Source: CAD feature listing. Evaluate the final solid. Frame: model axes, mm. Face numbers are marked on the shaded views. A direction names the side the tool comes from. Give positions to 0.01 mm unless a question says otherwise; leave off trailing zeros. Write each loop counter-clockwise with the first axis right and the second up, starting at its lowest first coordinate (ties: lowest second). Pieces come first, ordered by that corner, then holes. Notation, with made-up numbers: (43.5, 17.25) -> (69.5, 17.25) arc R24 ccw to (69.5, 48.25) -> close; hole circle Ø2 at (-28, 47.25). An arc over 180 degrees is marked (long way). Write item = value, one per line.
Autodesk Inventor part; units mm, degrees
ref_plane "YZ Plane" through (0, 0, 0) normal (1, 0, 0) x (0, 1, 0)
ref_plane "XZ Plane" through (0, 0, 0) normal (0, 1, 0) x (-1, 0, 0)
ref_plane "XY Plane" through (0, 0, 0) normal (0, 0, 1) x (1, 0, 0)
sketch "Sketch1" plane through (0, 0, 0) normal (0, 0, 1) x (1, 0, 0)
  circle A0 centre (0, 0) radius 1.7526
  dimension "d0" = 3.5052
extrude "Extrusion1" add sketch "Sketch1" along normal blind 31.75
sketch "Sketch2" plane through (0, 0, 0) normal (0, 0, -1) x (-1, 0, 0)
  circle A0 centre (0, 0) radius 1.7526 construction
  circle A1 centre (0, 0) radius 2.8702
  dimension "d3" = 5.7404
extrude "Extrusion2" add sketch "Sketch2" along normal blind 3.5052
sketch "Sketch3" plane through (0, 0, -3.5052) normal (0, 0, -1) x (-1, 0, 0)
  circle A0 centre (0, 0) radius 2.8702
  line L0 (0, 1.604) -> (1.3891, 0.802)
  line L1 (1.3891, 0.802) -> (1.3891, -0.802)
  line L2 (1.3891, -0.802) -> (0, -1.604)
  line L3 (0, -1.604) -> (-1.3891, -0.802)
  line L4 (-1.3891, -0.802) -> (-1.3891, 0.802)
  line L5 (-1.3891, 0.802) -> (0, 1.604)
  dimension "d6" = 2.7781
extrude "Extrusion3" cut sketch "Sketch3" against normal blind 1.7526 contours L0 L1 L2 L3 L4 L5
chamfer "Chamfer1" distance 0.508 angle 45 1 edges at (-1.7526, 0, 31.75)
thread "Thread2"
properties part number "6-32 SHCS x1250" material "Stainless Steel"
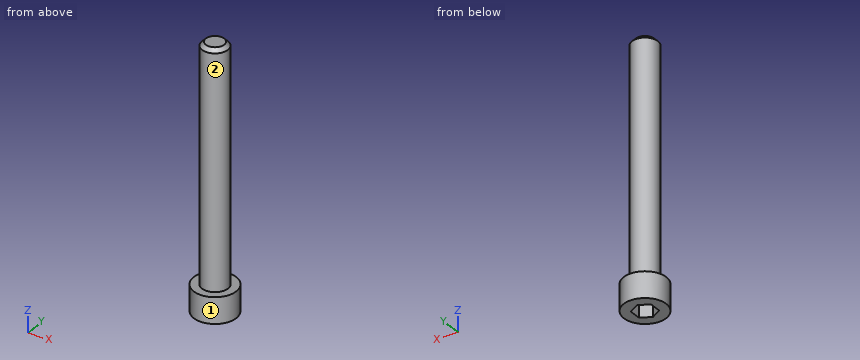
(1) Section query A-A (y = 0). Return loops of the section in (x, z).
Values follow:
outline = (-2.87, -3.51) -> (-1.39, -3.51) -> (-1.39, -1.75) -> (1.39, -1.75) -> (1.39, -3.51) -> (2.87, -3.51) -> (2.87, 0) -> (1.75, 0) -> (1.75, 31.24) -> (1.24, 31.75) -> (-1.24, 31.75) -> (-1.75, 31.24) -> (-1.75, 0) -> (-2.87, 0) -> close
(2) Access query for the marked faces 1 and 2. Directions: +Z, -Z, +X, -X, +Y, -Y. A direction counts if a zero-diameter tool reaches every point of the face in a straight line with its end or side. Return the directions, or none.
Values follow:
face_1 = +Z, -Z
face_2 = +Z
(3) First-contact query: pin 1 (0.8 mm diameter, centred on x = 0.5, y = 0.5, fed in from -Z); pin 2 (1.5 mm diameter, centred on y = 2, z = 11.5, fed in from -X); pin 3 (1 mm diameter, centred on y = -0.5, z = 6, fed in from -X). Flat tips, straight axial feed; report the tip coordinate or a pass-through.
Values follow:
pin_1 = -1.75
pin_2 = -1.23
pin_3 = -1.75
(4) Section query B-B (z = 11). Return loops of the section in (x, y).
Values follow:
outline = circle Ø3.51 at (0, 0)
(5) Section query C-C (x = 2.2). Return loops of the section in (y, z), plus the area to 3 significant figures.
Values follow:
outline = (-1.84, -3.51) -> (1.84, -3.51) -> (1.84, 0) -> (-1.84, 0) -> close
area = 12.9 mm2
(6) Material intervals for line 1 (Z direction, x = -2.2, y = -1.35); line 2 (X direction, y = 0.7, z = 28.5); line 3 (Z direction, x = 0.4, y = -0.75), sorted ascending.
Values follow:
line_1 = -3.51 to 0
line_2 = -1.61 to 1.61
line_3 = -1.75 to 31.75
